from build123d import *

# Parameters (mm, degrees)
F0_R     = 12.7
F1_DEPTH = 38.1
F2_R     = 1.651
F3_DEPTH = 12.7
F4_R     = 5.08
F5_SIZE  = 0.508


with BuildPart() as f1:
    # F0 (on Front) → F1 (new body, symmetric)
    with BuildSketch(Plane.XZ):
        with BuildLine():
            Line((19.05, -25.4), (19.05, 0))
            ThreePointArc((19.05, 0), (0, 19.05), (-19.05, 0))
            Line((-19.05, 0), (-19.05, -25.4))
            Line((-19.05, -25.4), (19.05, -25.4))
        make_face()
        Circle(F0_R, mode=Mode.SUBTRACT)
    extrude(amount=F1_DEPTH, both=True)

    # F2 (on face) → F3 (cut)
    with BuildSketch(Plane(origin=(0, 0, -25.4), x_dir=(1, 0, 0), z_dir=(0, 0, -1))):
        with Locations((-12.7, 31.75)):
            Circle(F2_R)
        with Locations((11.049, 31.75)):
            Circle(F2_R)
        with Locations((-12.7, -31.75)):
            Circle(F2_R)
        with Locations((11.049, -31.75)):
            Circle(F2_R)
    extrude(amount=-F3_DEPTH, mode=Mode.SUBTRACT)

    # F4
    f4_edges = [f1.edges().sort_by_distance(p)[0] for p in [
        (0, 38.1, 19.05),
        (0, -38.1, 19.05),
    ]]
    fillet(f4_edges, radius=F4_R)

    # F5
    f5_edges = [f1.edges().sort_by_distance(p)[0] for p in [
        (-12.7, 38.1, 0),
        (-12.7, -38.1, 0),
    ]]
    chamfer(f5_edges, length=F5_SIZE)


solid = f1.part
Could you check a few things on this model? Use its own coordinates, in mm. A direction names the side the tool comes from. Round coordinates to 2 decimals unless told otherwise and drop trailing zeros. Order: outer loops, then holes, each group sorted by start corner. A loop starts at its lowest first (then second) coordinate and runs counter-clockwise, first axis right, second up.
Q1. Imagine slicing it at C-C, the plane y = 2. List the corners of the cut face in (x, z) for me, then the cut area to 3 significant figures.
Geometry says:
outline: (-19.05, -25.4) - (19.05, -25.4) - (19.05, 0) arc R19.05 ccw to (-19.05, 0) - close; hole circle Ø25.4 at (0, 0)
area: 1,030 mm2
Q2. Imagine slicing it at B-B, the plane y = 31.75. List the corners of the cut face in (x, z) for me, then the cut area to 3 significant figures.
Geometry says:
outline: (-19.05, -25.4) - (-14.35, -25.4) - (-14.35, -12.7) - (-11.05, -12.7) - (-11.05, -25.4) - (9.4, -25.4) - (9.4, -12.7) - (12.7, -12.7) - (12.7, -25.4) - (19.05, -25.4) - (19.05, 0) arc R19.05 ccw to (-19.05, 0) - close; hole circle Ø25.4 at (0, 0)
area: 947 mm2
Q3. I'm going to push flat-ended pins straight in: P1, Ø1, axis at x = 11.5, y = -32, coming from the -Z side; P2, Ø5, axis at y = -12, z = 3.5, coming from the +X side; P3, Ø5, axis at x = -5, y = -10.5, coming from the +Z side. Where does each tip first touch, or does it pass through?
Geometry says:
P1: stops at z = -12.7
P2: stops at x = 19.02
P3: stops at z = 18.89
Q4. Thinking about a two-plate mould opening in Y: for faces 1 (the face through (-2.75, 0.53, -12.4)), 2 (the face through (11.94, 30.36, -19.14)), 3 (the face through (-17.522, 36.651, -12.878)), which applies, released by +Y, released by -Y, zero draft, split by the parting line, or undercut?
Geometry says:
face 1: zero draft
face 2: undercut
face 3: released by +Y
Q5. Please list where these lines run through material, in increasing order: probe 1 along X at (y, z) = (31.75, -21.75); probe 2 along Y at (x, z) = (-12.7, -21.5); probe 3 along X at (y, z) = (31.5, -0.5).
Geometry says:
probe 1: x = -19.05 to -14.35, -11.05 to 9.4, 12.7 to 19.05
probe 2: y = -38.1 to -33.4, -30.1 to 30.1, 33.4 to 38.1
probe 3: x = -19.05 to -12.69, 12.69 to 19.05
Q6. Imagine slicing it at A-A, the plane x = 0. List the corners of the cut face in (y, z) for me.
Geometry says:
outline: (-38.1, -25.4) - (38.1, -25.4) - (38.1, -13.21) - (37.59, -12.7) - (-37.59, -12.7) - (-38.1, -13.21) - close; (-38.1, 13.21) - (-37.59, 12.7) - (37.59, 12.7) - (38.1, 13.21) - (38.1, 13.97) arc R5.08 ccw to (33.02, 19.05) - (-33.02, 19.05) arc R5.08 ccw to (-38.1, 13.97) - close
Q7. Which directions (+Z, -Z, +X, -X, +Y, -Y) give clear straight access to the entire face, cutting with the end or side of a thin tool? Please do faces 4 (the face through (-19.05, 0, -13)), 5 (the face through (-11.81, -33.14, -19.14)).
Geometry says:
face 4: +Z, -Z, -X, +Y, -Y
face 5: -Z
